```python
from build123d import *

# Parameters (mm, degrees)
F0_W     = 15
F0_H     = 15
F1_DEPTH = 15
F2_R     = 2.5
F3_DEPTH = 7
F4_W     = 12
F4_H     = 12
F5_DEPTH = 13
F6_R     = 3
F7_DEPTH = 5


with BuildPart() as f1:
    # F0 (on Top) → F1 (new body)
    with BuildSketch(Plane.XY):
        Rectangle(F0_W, F0_H)
    extrude(amount=F1_DEPTH)

    # F2 (on face) → F3 (join)
    with BuildSketch(Plane.XY.offset(15)):
        Circle(F2_R)
    extrude(amount=F3_DEPTH)

    # F4 (on face) → F5 (cut)
    with BuildSketch(Plane(origin=(0, 0, 0), x_dir=(1, 0, 0), z_dir=(0, 0, -1))):
        Rectangle(F4_W, F4_H)
    extrude(amount=-F5_DEPTH, mode=Mode.SUBTRACT)

    # F6 (on face) → F7 (join)
    with BuildSketch(Plane(origin=(0, 0, 13), x_dir=(1, 0, 0), z_dir=(0, 0, -1))):
        Circle(F6_R)
    extrude(amount=F7_DEPTH)


solid = f1.part
```
Model file for the job. Use its own axes, mm. A direction names the side the tool comes from. Coordinates: 2 decimals unless noted, no trailing zeros. Loops run counter-clockwise (first coordinate to the right, second up) from the corner with the lowest first, then second, coordinate; pieces in that order, holes last. Notation, with made-up numbers: M -4.75,-13 L 51.25,-13 A34 ccw 51.25,18 Z; hole C -2,14 d8. An arc over 180 degrees is marked long. Use CSV: the item, a comma, the result in double quotes. Start each with the question number.
1. Tool access for faces 4 (the cylindrical face through (-0.54, -2.44, 18.45)), 5 (the flat face through (0, 0, 22)), 6 (the flat face through (6, 0, 6)): list every direction of +Z, -Z, +X, -X, +Y, -Y with a clear straight run to the whole face (end or side of a thin tool).
2. Two-plate mould, pull along Y, no slides. Class faces 1 (the flat face through (0, 7.5, 7)), 2 (the flat face through (-7.5, 0, 7)), 3 (the flat face through (0, 0, 8)): pulls with the +Y half, pulls with the -Y half, needs draft (parallel to the pull), parting line crosses it, or undercut.
3. Band-saw the part on D-D, the plane y = -4.75. List the corners of the cut face in (x, z), then the cut area to 3 significant figures.
4. Band-saw the part on A-A, the plane z = 12.75. List the corners of the cut face in (x, y).
5. Probe probe 1 along X at (y, z) = (1, 6); probe 2 along X at (y, z) = (1.5, 11). List the from-to ranges inside material, lowest first. Write a range as [from, to].
6. Flat gauge pins, fed straight in: pin 1 (3 mm diameter, centred on x = 0, y = 5.5, fed in from +Z); pin 2 (6.5 mm diameter, centred on x = 1.5, y = 0, fed in from -Z). Where does each tip first touch, or does it go through?
7. Band-saw the part on B-B, the plane y = 0. List the corners of the cut face in (x, z), then the cut area to 3 significant figures.
Entries:
1,face 4,"+Z"
1,face 5,"+Z, +X, -X, +Y, -Y"
1,face 6,"-Z"
2,face 1,"pulls with the +Y half"
2,face 2,"needs draft"
2,face 3,"undercut"
3,outline,"M -7.5,0 L -6,0 L -6,13 L 6,13 L 6,0 L 7.5,0 L 7.5,15 L -7.5,15 Z"
3,area,"69.0 mm2"
4,outline,"M -7.5,-7.5 L 7.5,-7.5 L 7.5,7.5 L -7.5,7.5 Z; C 0,0 d6; hole M -6,-6 L 6,-6 L 6,6 L -6,6 Z"
5,probe 1,"x = [-7.5, -6], [6, 7.5]"
5,probe 2,"x = [-7.5, -6], [-2.6, 2.6], [6, 7.5]"
6,pin 1,"stops at z = 15"
6,pin 2,"stops at z = 8"
7,outline,"M -7.5,0 L -6,0 L -6,13 L -3,13 L -3,8 L 3,8 L 3,13 L 6,13 L 6,0 L 7.5,0 L 7.5,15 L 2.5,15 L 2.5,22 L -2.5,22 L -2.5,15 L -7.5,15 Z"
7,area,"134 mm2"
